Model file for the job. Use its own axes, mm. Face numbers are marked on the shaded views. Coordinates: 2 decimals unless noted, no trailing zeros. Order: outer loops, then holes, each group sorted by start corner. A loop starts at its lowest first (then second) coordinate and runs counter-clockwise, first axis right, second up.
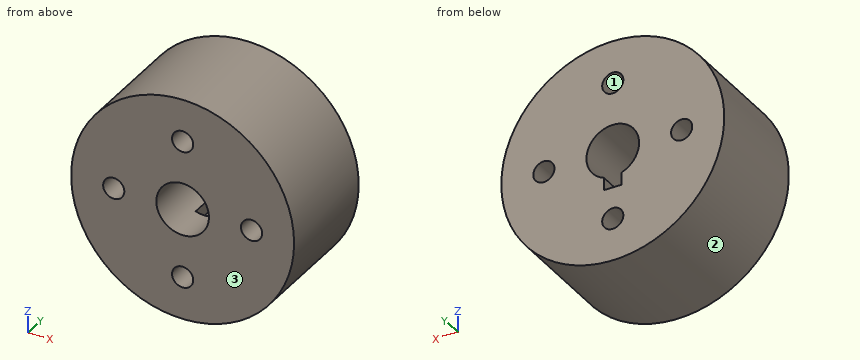
from build123d import *

# Parameters (mm, degrees)
SKETCH1_R           = 25.4
SKETCH1_R_2         = 6
BOSS_EXTRUDE1_DEPTH = 25.4
SKETCH2_W           = 4
SKETCH2_H           = 5
CUT_EXTRUDE1_DEPTH  = 16.825
SKETCH3_R           = 2.413
CUT_EXTRUDE2_DEPTH  = 26.4


with BuildPart() as part:
    # Sketch1 → Boss-Extrude1 (new body)
    with BuildSketch(Plane(origin=(0, 0, 0), x_dir=(1, 0, 0), z_dir=(0, 1, 0))):
        Circle(SKETCH1_R)
        Circle(SKETCH1_R_2, mode=Mode.SUBTRACT)
    extrude(amount=BOSS_EXTRUDE1_DEPTH)

    # Sketch2 → Cut-Extrude1 (cut)
    with BuildSketch(Plane(origin=(0, 25.4, 0), x_dir=(1, 0, 0), z_dir=(0, 1, 0))):
        with Locations((0, 6)):
            Rectangle(SKETCH2_W, SKETCH2_H)
    extrude(amount=-CUT_EXTRUDE1_DEPTH, mode=Mode.SUBTRACT)

    # Sketch3 → Cut-Extrude2 (cut, through all)
    with BuildSketch(Plane.XZ):
        with Locations((0, -15.7)):
            Circle(SKETCH3_R)
        with Locations((-15.7, 0)):
            Circle(SKETCH3_R)
        with Locations((0, 15.7)):
            Circle(SKETCH3_R)
        with Locations((15.7, 0)):
            Circle(SKETCH3_R)
    extrude(amount=-CUT_EXTRUDE2_DEPTH, mode=Mode.SUBTRACT)


solid = part.part
Q1. Cut at C-C, the plane x = 14.5. List the corners of the cut face in (y, z), plus the area to 3 significant figures.
Established:
outline: (0, -20.85) - (25.4, -20.85) - (25.4, -2.09) - (0, -2.09) - close; (0, 2.09) - (25.4, 2.09) - (25.4, 20.85) - (0, 20.85) - close
area: 953 mm2
Q2. Drop flat-ended pins along their axis: P1, Ø1.4, axis at y = 17, z = -7, coming from the -X side; P2, Ø1.4, axis at x = -1, z = -7, coming from the +Y side (3 decimals); P3, Ø1.2, axis at x = 1, y = 20.5, coming from the +Z side; P4, Ø3, axis at x = 15.7, z = 0, coming from the -Y side. Give the stop position or say it passes through.
Established:
P1: stops at x = -24.61
P2: stops at y = 8.575
P3: stops at z = 25.4
P4: passes through
Q3. Cut at B-B, the plane z = -14. List the corners of the cut face in (x, y), plus the area to 3 significant figures.
Established:
outline: (-21.19, 0) - (-1.71, 0) - (-1.71, 25.4) - (-21.19, 25.4) - close; (1.71, 0) - (21.19, 0) - (21.19, 25.4) - (1.71, 25.4) - close
area: 990 mm2
Q4. Cut at D-D, the plane y = 3. List the corners of the cut face in (x, z).
Established:
outline: circle Ø50.8 at (0, 0); hole circle Ø4.83 at (-15.7, 0); hole circle Ø12 at (0, 0); hole circle Ø4.83 at (0, -15.7); hole circle Ø4.83 at (0, 15.7); hole circle Ø4.83 at (15.7, 0)
Q5. Cut at A-A, the plane y = 20. List the corners of the cut face in (x, z).
Established:
outline: circle Ø50.8 at (0, 0); hole circle Ø4.83 at (-15.7, 0); hole circle Ø4.83 at (0, -15.7); hole circle Ø4.83 at (0, 15.7); hole (-2, -8.5) - (2, -8.5) - (2, -5.66) arc R6 ccw (long way) to (-2, -5.66) - close; hole circle Ø4.83 at (15.7, 0)
Q6. Probe line 1 (Z direction, x = 0, y = 13.25); line 2 (Z direction, x = 5.5, y = 10); line 3 (X direction, y = 12.25, z = 0.5). List the from-to ranges inside material, lowest first.
Established:
line 1: z = -25.4 to -18.11, -13.29 to -8.5, 6 to 13.29, 18.11 to 25.4
line 2: z = -24.8 to -2.4, 2.4 to 24.8
line 3: x = -25.4 to -18.06, -13.34 to -5.98, 5.98 to 13.34, 18.06 to 25.4
Q7. Mould opens along X. For the marked faces 1, 2 and 3 say: pulls with the +X half, pulls with the -X half, needs draft (parallel to the pull), parting line crosses it, or undercut.
Established:
face 1: undercut
face 2: parting line crosses it
face 3: needs draft
